```python
from build123d import *

# Parameters (mm, degrees)
SKETCH1_R           = 19.05
BOSS_EXTRUDE1_DEPTH = 6.35
BOSS_EXTRUDE1_DRAFT = -1
CUT_EXTRUDE3_DEPTH  = 20.05
CIRPATTERN3_COUNT   = 24
SKETCH7_R           = 19.05
SKETCH7_R_2         = 16.637
BOSS_EXTRUDE3_DEPTH = 6.35
BOSS_EXTRUDE3_DRAFT = -1
FILLET2_R           = 0.762


with BuildPart() as part:
    # Sketch1 → Boss-Extrude1 (with draft: the straight prism first)
    with BuildSketch(Plane(origin=(0, 0, 0), x_dir=(1, 0, 0), z_dir=(0, 1, 0))):
        Circle(SKETCH1_R)
    extrude(amount=-BOSS_EXTRUDE1_DEPTH)
    # Boss-Extrude1: the draft: its side faces are tilted about the plane it starts from
    boss_extrude1_sides = [part.faces().sort_by_distance(p)[0] for p in [
        (-19.05, -3.175, 0),
    ]]
    draft(boss_extrude1_sides, Plane(origin=(0, 0, 0), x_dir=(1, 0, 0), z_dir=(0, 1, 0)), BOSS_EXTRUDE1_DRAFT)

    # Sketch6 → Cut-Extrude3 (cut, through all)
    with BuildSketch(Plane.XY):
        Polygon((0, -2.54), (-6.985, -9.525), (6.985, -9.525), align=None)
    cut_extrude3 = extrude(amount=-CUT_EXTRUDE3_DEPTH, mode=Mode.SUBTRACT)

    # CirPattern3: Cut-Extrude3 ×24 about axis
    cirpattern3_axis = Axis((0, 0, 0), (0, 1, 0))
    for i in range(1, CIRPATTERN3_COUNT):
        add(cut_extrude3.rotate(cirpattern3_axis, i * 360 / CIRPATTERN3_COUNT), mode=Mode.SUBTRACT)


with BuildPart() as boss_extrude3_tool:
    # Sketch7 → Boss-Extrude3 (with draft: the straight prism first)
    with BuildSketch(Plane(origin=(0, 0, 0), x_dir=(1, 0, 0), z_dir=(0, 1, 0))):
        Circle(SKETCH7_R)
        Circle(SKETCH7_R_2, mode=Mode.SUBTRACT)
    extrude(amount=-BOSS_EXTRUDE3_DEPTH)
    # Boss-Extrude3: the draft: its side faces are tilted about the plane it starts from
    boss_extrude3_sides = [boss_extrude3_tool.faces().sort_by_distance(p)[0] for p in [
        (-19.05, -3.175, 0),
        (-16.637, -3.175, 0),
    ]]
    draft(boss_extrude3_sides, Plane(origin=(0, 0, 0), x_dir=(1, 0, 0), z_dir=(0, 1, 0)), BOSS_EXTRUDE3_DRAFT)


with BuildPart() as part_1:
    add(part.part)

    # Boss-Extrude3: add boss_extrude3_tool
    add(boss_extrude3_tool.part)

    # Fillet2
    fillet2_edges = [part_1.edges().sort_by_distance(p)[0] for p in [
        (-18.939160338, -6.35, 0),
        (-16.747839662, -6.35, 0),
    ]]
    fillet(fillet2_edges, radius=FILLET2_R)


solid = part_1.part
```
Can you work these out from the model? Positions are in its coordinate system, mm. Coordinates: 2 decimals unless noted, no trailing zeros. Order: outer loops, then holes, each group sorted by start corner. A loop starts at its lowest first (then second) coordinate and runs counter-clockwise, first axis right, second up.
1. I need wall thicknesses on line 1 (Z direction, x = 2.5, y = -4.75); line 2 (Z direction, x = -6.5, y = -5.25); line 3 (X direction, y = -5, z = 6). Which ranges of each line are inside material? Lowest first, please.
2. Thinking about a two-plate mould opening in Z: for faces 1 (the face through (-4.12, -3.38, 18.54)), 2 (the face through (-6.538, -3.373, 7.716)), 3 (the face through (0, 0, 0)), which applies, +Z half, -Z half, draft (parallel to the pull), parting line (faces both ways), or undercut?
3. I'm going to push flat-ended pins straight in: pin 1 (5 mm diameter, centred on x = -10.5, z = 10.5, fed in from +Y); pin 2 (2 mm diameter, centred on x = -10, y = -4, fed in from +Z). Where does each tip first touch, or does it pass through?
4. If we section it at A-A (y = -1.75): Please give me the cut outline in (x, z), then the cut area to 3 significant figures.
Entries:
1. line 1: z = -18.8 to -16.53, 16.53 to 18.8
1. line 2: z = -17.81 to -15.41, 15.41 to 17.81
1. line 3: x = -17.99 to -15.61, 15.61 to 17.99
2. face 1: parting line
2. face 2: undercut
2. face 3: draft
3. pin 1: stops at y = 0
3. pin 2: stops at z = 16.71
4. outline: circle Ø38.04 at (0, 0)
4. area: 1,140 mm2
